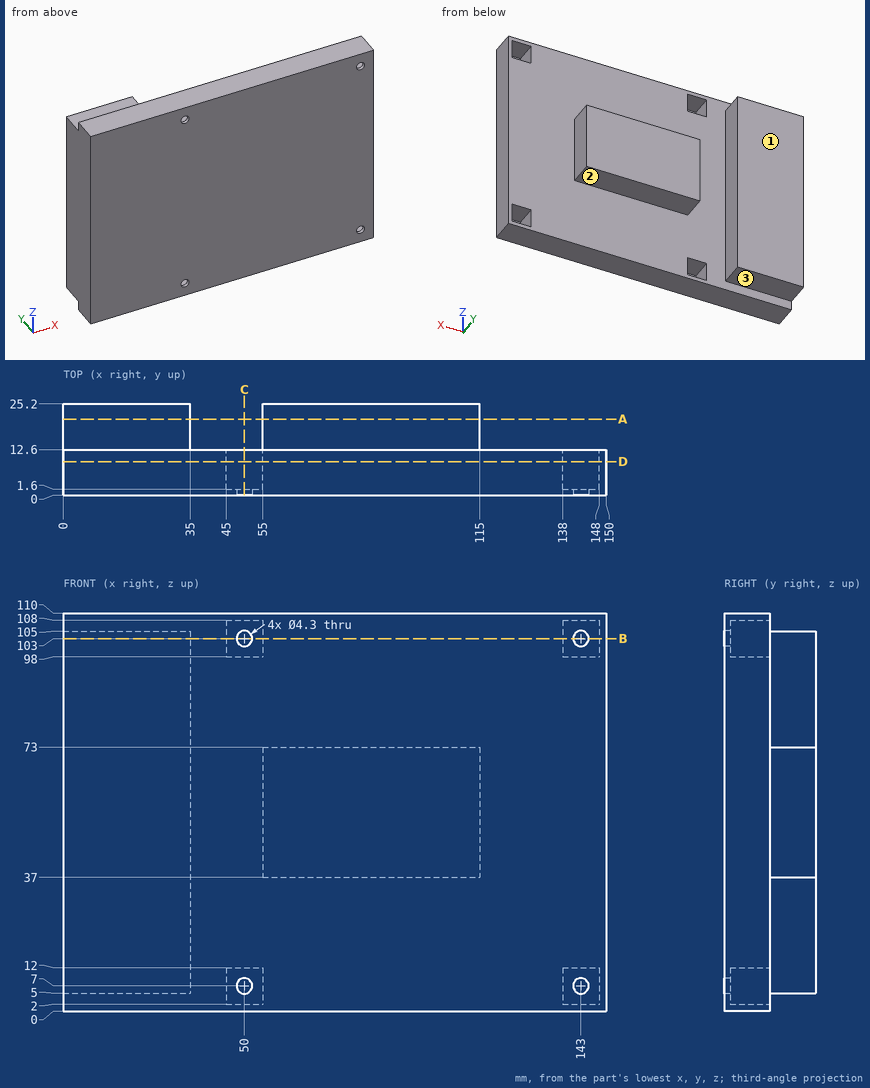
Here's the drawing with two shaded views (mm, measured from the low corner). I have some questions. A direction names the side the tool comes from. Give positions to 0.01 mm unless a question says otherwise; leave off trailing zeros. Order: outer loops, then holes, each group sorted by start corner. A loop starts at its lowest first (then second) coordinate and runs counter-clockwise, first axis right, second up. Notation, with made-up numbers: M 0,43 L 21,43 A12 cw 21,63 Z; hole C 38.5,56.25 d8. An arc over 180 degrees is marked long. One line per item, written item: value.
1) For P1, Ø14, axis at x = 81, y = 20.5, coming from the +Z side; P2, Ø6.5, axis at x = 15.5, y = 19.5, coming from the -Z side; P3, Ø5.5, axis at x = 50, z = 103, coming from the +Y side, each with a flat end and sliding along its axis, tell me the tip position at first contact or that it passes through.
Answer sheet:
P1: stops at z = 73
P2: stops at z = 5
P3: stops at y = 1.6
2) I want a section at A-A, the plane y = 21. List the corners of the cut face in (x, z) for me, plus the area to 3 significant figures.
Answer sheet:
outline: M 0,5 L 35,5 L 35,105 L 0,105 Z; M 55,37 L 115,37 L 115,73 L 55,73 Z
area: 5,660 mm^2
3) On a 3-axis mill with a long thin cutter (end or side, diameter ignored), from which of +Z, -Z, +X, -X, +Y, -Y can I reach the whole of each face in a straight line? I mean the marked faces 1, 2 and 3. Say none if no direction works.
Answer sheet:
face 1: +Z, -Z, +X, -X, +Y
face 2: -Z, +X, +Y
face 3: -Z, +X, -X, +Y
4) Please list where these lines run through material, in increasing order: line 1 along Z through (x, y) = (143, 0.4); line 2 along X through (y, z) = (0.4, 103); line 3 along Z through (x, y) = (46.5, 10.25).
Answer sheet:
line 1: z = 0 to 4.85, 9.15 to 100.85, 105.15 to 110
line 2: x = 0 to 47.85, 52.15 to 140.85, 145.15 to 150
line 3: z = 0 to 2, 12 to 98, 108 to 110
5) I want a section at C-C, the plane x = 50. List the corners of the cut face in (y, z) for me.
Answer sheet:
outline: M 0,0 L 12.6,0 L 12.6,2 L 1.6,2 L 1.6,4.85 L 0,4.85 Z; M 0,9.15 L 1.6,9.15 L 1.6,12 L 12.6,12 L 12.6,98 L 1.6,98 L 1.6,100.85 L 0,100.85 Z; M 0,105.15 L 1.6,105.15 L 1.6,108 L 12.6,108 L 12.6,110 L 0,110 Z
6) I want a section at B-B, the plane z = 103. List the corners of the cut face in (x, y) for me, plus the area to 3 significant figures.
Answer sheet:
outline: M 0,0 L 47.85,0 L 47.85,1.6 L 45,1.6 L 45,12.6 L 35,12.6 L 35,25.2 L 0,25.2 Z; M 52.15,0 L 140.85,0 L 140.85,1.6 L 138,1.6 L 138,12.6 L 55,12.6 L 55,1.6 L 52.15,1.6 Z; M 145.15,0 L 150,0 L 150,12.6 L 148,12.6 L 148,1.6 L 145.15,1.6 Z
area: 2,100 mm^2
7) I want a section at D-D, the plane y = 9.25. List the corners of the cut face in (x, z) for me, plus the area to 3 significant figures.
Answer sheet:
outline: M 0,0 L 150,0 L 150,110 L 0,110 Z; hole M 45,2 L 55,2 L 55,12 L 45,12 Z; hole M 45,98 L 55,98 L 55,108 L 45,108 Z; hole M 138,2 L 148,2 L 148,12 L 138,12 Z; hole M 138,98 L 148,98 L 148,108 L 138,108 Z
area: 16,100 mm^2
